```python
from build123d import *

# Parameters (mm, degrees)
ESBO_O1_R                  = 12.85
ESBO_O1_R_2                = 11.35
RESSALTO_EXTRUS_O1_DEPTH   = 35
ESBO_O2_R                  = 12.85
RESSALTO_EXTRUS_O2_DEPTH   = 1.5
ESBO_O3_W                  = 3
ESBO_O3_H                  = 3
CORTE_EXTRUS_O1_DEPTH      = 13.85
CORTE_EXTRUS_O1_DEPTH_BACK = 13.85


with BuildPart() as part:
    # Esboço1 → Ressalto-extrusão1 (new body)
    with BuildSketch(Plane.XY):
        Circle(ESBO_O1_R)
        Circle(ESBO_O1_R_2, mode=Mode.SUBTRACT)
    extrude(amount=RESSALTO_EXTRUS_O1_DEPTH)

    # Esboço2 → Ressalto-extrusão2 (add)
    with BuildSketch(Plane(origin=(0, 0, 0), x_dir=(-1, 0, 0), z_dir=(0, 0, -1))):
        Circle(ESBO_O2_R)
    extrude(amount=RESSALTO_EXTRUS_O2_DEPTH)

    # Esboço3 → Corte-extrusão1 (cut, two sides)
    with BuildSketch(Plane(origin=(0, 0, 0), x_dir=(1, 0, 0), z_dir=(0, 1, 0))) as corte_extrus_o1_sk:
        with Locations((0, -32)):
            Rectangle(ESBO_O3_W, ESBO_O3_H)
    extrude(amount=CORTE_EXTRUS_O1_DEPTH, mode=Mode.SUBTRACT)
    extrude(corte_extrus_o1_sk.sketch, amount=-CORTE_EXTRUS_O1_DEPTH_BACK, mode=Mode.SUBTRACT)


solid = part.part
```
Here's how the part is built. I have some questions about the finished solid (model axes, mm). A direction names the side the tool comes from. Give positions to 0.01 mm unless a question says otherwise; leave off trailing zeros. Loops run counter-clockwise (first coordinate to the right, second up) from the corner with the lowest first, then second, coordinate; pieces in that order, holes last. Notation, with made-up numbers: M -9,22 L 5,22 A8 cw 5,31 Z; hole C -25,-38.5 d8. An arc over 180 degrees is marked long. Put each result on its own line as item: value. Start each with the question number.
(1) I want a section at D-D on x = -4.75. Please give me the cut outline in (y, z), then the cut area to 3 significant figures.
(2) Will these pins go through, and if not, where does the flat tip stop? pin 1 Ø0.5 at (y, z) = (12, 32.5) entering from -X; pin 2 Ø1.7 at (y, z) = (-12, 32.5) entering from -X; pin 3 Ø0.5 at (y, z) = (12, 32) entering from +X.
(3) For faces 1 (the flat face through (0, -12, 30.5)), 2 (the flat face through (0, 0, -1.5)), 3 (the cylindrical face through (5.24, -10.07, 17.26)), which set-ups out of +Z, -Z, +X, -X, +Y, -Y let a thin tool reach every point of the face, with its end or its side?
(4) If we mould it in two halves opening along Y, with no side actions, what happens to faces 4 (the flat face through (0, 0, 0)), 5 (the flat face through (1.5, -12, 32))? For each: +Y half, -Y half, draft (parallel to the pull), parting line (faces both ways), or undercut.
(5) I want a section at B-B on y = 0. Please give me the cut outline in (x, z).
(6) I need wall thicknesses on line 1 along Y through (x, z) = (0, 24.5); line 2 along Z through (x, y) = (-2, 9.5); line 3 along X through (y, z) = (-4.75, 14). Which ranges of each line are inside material? Lowest first, please. Write a range as [from, to].
(7) I want a section at C-C on z = 20.5. Please give me the cut outline in (x, y).
(8) I want a section at A-A on x = 0. Please give me the cut outline in (y, z).
Answer block:
1. outline: M -11.94,-1.5 L 11.94,-1.5 L 11.94,35 L 10.31,35 L 10.31,0 L -10.31,0 L -10.31,35 L -11.94,35 Z
1. area: 150 mm^2
2. pin 1: x = -5.2
2. pin 2: x = -6.39
2. pin 3: x = 5.2
3. face 1: +Y, -Y
3. face 2: -Z, +X, -X, +Y, -Y
3. face 3: +Z
4. face 4: undercut
4. face 5: draft
5. outline: M -12.85,-1.5 L 12.85,-1.5 L 12.85,35 L 11.35,35 L 11.35,0 L -11.35,0 L -11.35,35 L -12.85,35 Z
6. line 1: [-12.85, -11.35], [11.35, 12.85]
6. line 2: [-1.5, 0]
6. line 3: [-11.94, -10.31], [10.31, 11.94]
7. outline: C 0,0 d25.7; hole C 0,0 d22.7
8. outline: M -12.85,-1.5 L 12.85,-1.5 L 12.85,30.5 L 11.35,30.5 L 11.35,0 L -11.35,0 L -11.35,30.5 L -12.85,30.5 Z; M -12.85,33.5 L -11.35,33.5 L -11.35,35 L -12.85,35 Z; M 11.35,33.5 L 12.85,33.5 L 12.85,35 L 11.35,35 Z
